Check sheet for the modelled part. Datum: model origin and axes. Units: mm. Face numbers are marked on the shaded views. A direction names the side the tool comes from. Coordinates: 2 decimals unless noted, no trailing zeros. Loops run counter-clockwise (first coordinate to the right, second up) from the corner with the lowest first, then second, coordinate; pieces in that order, holes last. Notation, with made-up numbers: (-6.5, -2.5) - (7.5, -2.5) arc R15 ccw to (7.5, 6.5) - close; hole circle Ø2 at (72, -1.75). An arc over 180 degrees is marked (long way). Use a Markdown table: item, result. Add a question column.
1) Sectioned sample at B-B, the plane z = 280. Enter the section's corners in (x, y).
2) Thickness scan on line 1 (Z direction, x = 16, y = -125); line 2 (X direction, y = -239.5, z = 49); line 3 (Z direction, x = 39, y = -97.5). Record the ranges inside material, lowest first.
3) Sectioned sample at D-D, the plane x = 50.5. Enter the section's corners in (y, z).
4) Go/stop test with flat-tipped pins: P1, Ø8, axis at y = -72, z = 65, coming from the -X side; P2, Ø4, axis at x = 59, y = -211, coming from the +Z side; P3, Ø6, axis at y = -75.5, z = 44.5, coming from the +X side. Record where each tip stops, or that it passes through.
5) Sectioned sample at C-C, the plane z = 111. Enter the section's corners in (x, y).
6) Tool access check on the marked faces 1 and 2. Record the directions out of +Z, -Z, +X, -X, +Y, -Y that give a thin tool (end or side, any length) a straight path to the whole face; none if there is none.
7) Draft check along Y on the marked faces 3 and 4. Enter one of: pulls with the +Y half, pulls with the -Y half, needs draft (parallel to the pull), parting line crosses it, or undercut.
8) Sectioned sample at A-A, the plane y = -125. Enter the section's corners in (x, z).
from build123d import *

# Parameters (mm, degrees)
F0_W     = 50
F0_H     = 25
F1_DEPTH = 250
F3_D     = 140
F3_DEPTH = 60
F4_R     = 100
F5_SIZE  = 5


with BuildPart() as f1:
    # F0 (on Front) → F1 (new body)
    with BuildSketch(Plane.XZ):
        Polygon((0, 25), (0, 0), (33, 0), (33, 25), (33, 400), (0, 400), align=None)
        with Locations((-25, 12.5)):
            Rectangle(F0_W, F0_H)
        with Locations((58, 12.5)):
            Rectangle(F0_W, F0_H)
    extrude(amount=F1_DEPTH)

    # F3
    with Locations(Plane.YZ.offset(33)):
        with Locations((-125, 280)):
            Hole(F3_D / 2, depth=F3_DEPTH)

    # F4
    f4_edges = [f1.edges().sort_by_distance(p)[0] for p in [
        (16.5, 0, 400),
        (16.5, -250, 400),
    ]]
    fillet(f4_edges, radius=F4_R)

    # F5
    f5_edges = [f1.edges().sort_by_distance(p)[0] for p in [
        (-50, -125, 25),
        (-50, -125, 0),
        (-50, 0, 12.5),
        (-50, -250, 12.5),
        (-25, -250, 25),
        (0, -250, 162.5),
        (33, -250, 162.5),
        (-25, 0, 25),
        (16.5, 0, 0),
        (58, 0, 25),
        (83, 0, 12.5),
        (83, -125, 25),
        (83, -125, 0),
        (83, -250, 12.5),
        (58, -250, 25),
        (16.5, -250, 0),
    ]]
    chamfer(f5_edges, length=F5_SIZE)


solid = f1.part
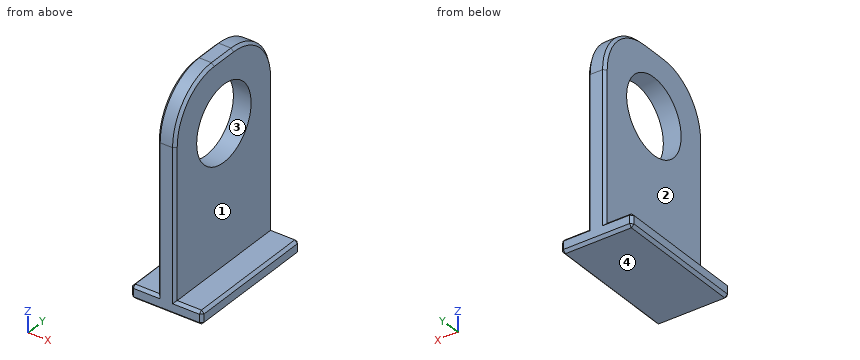
Solved:
| question | item | result |
|---|---|---|
| 1 | outline | (0, -245) - (5, -250) - (28, -250) - (33, -245) - (33, -195) - (0, -195) - close; (0, -55) - (33, -55) - (33, -5) - (28, 0) - (5, 0) - (0, -5) - close |
| 2 | line 1 | z = 0 to 210, 350 to 400 |
| 2 | line 2 | x = 0 to 33 |
| 2 | line 3 | z = 0 to 25 |
| 3 | outline | (-250, 5) - (-245, 0) - (-5, 0) - (0, 5) - (0, 20) - (-5, 25) - (-245, 25) - (-250, 20) - close |
| 4 | P1 | stops at x = 0 |
| 4 | P2 | stops at z = 25 |
| 4 | P3 | stops at x = 33 |
| 5 | outline | (0, -245) - (5, -250) - (28, -250) - (33, -245) - (33, -5) - (28, 0) - (5, 0) - (0, -5) - close |
| 6 | face 1 | +Z, +X, +Y, -Y |
| 6 | face 2 | +Z, -X, +Y, -Y |
| 7 | face 3 | undercut |
| 7 | face 4 | needs draft |
| 8 | outline | (-50, 5) - (-45, 0) - (78, 0) - (83, 5) - (83, 20) - (78, 25) - (33, 25) - (33, 210) - (0, 210) - (0, 25) - (-45, 25) - (-50, 20) - close; (0, 350) - (33, 350) - (33, 395) - (28, 400) - (5, 400) - (0, 395) - close |
